Could you check a few things on this drawing? It's one solid part, dimensions in mm from its lowest x, y, z. Round coordinates to 2 decimals unless told otherwise and drop trailing zeros. Write each loop counter-clockwise with the first axis right and the second up, starting at its lowest first coordinate (ties: lowest second). Pieces come first, ordered by that corner, then holes. Notation, with made-up numbers: (-31.75, 82) - (23.25, 82) arc R23 ccw to (23.25, 111) - close; hole circle Ø3 at (-13, 81). An arc over 180 degrees is marked (long way). Put each result on its own line as item: value.
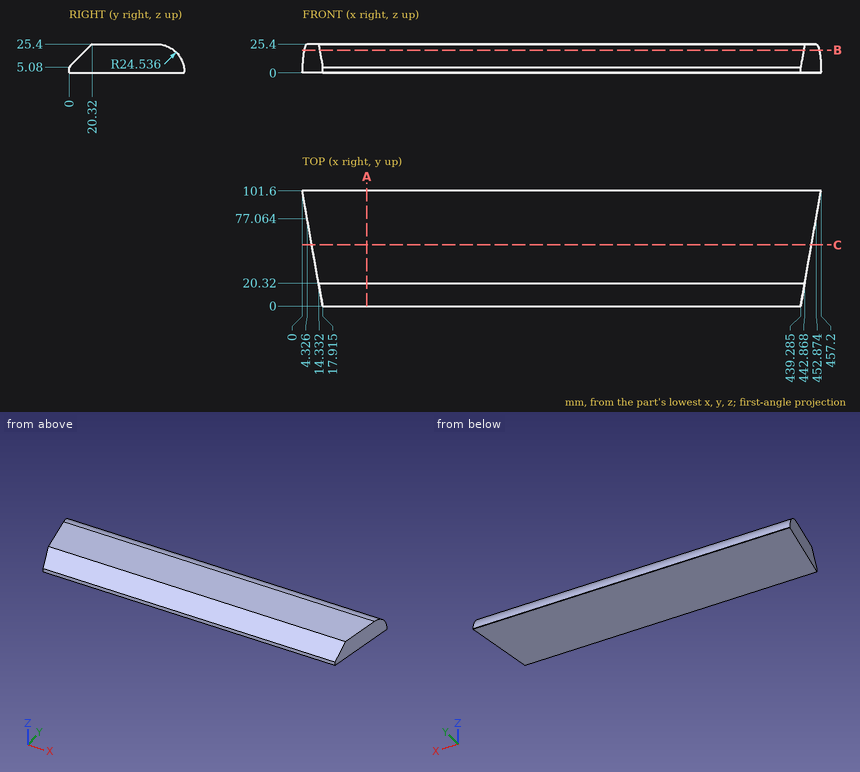
(1) Imagine slicing it at A-A, the plane x = 57. List the corners of the cut face in (y, z) for me.
Values found:
outline: (0, 0) - (101.6, 0) - (101.6, 0.86) arc R24.54 ccw to (77.06, 25.4) - (20.32, 25.4) - (0, 5.08) - close
(2) Imagine slicing it at B-B, the plane z = 20. List the corners of the cut face in (x, y) for me, then the cut area to 3 significant figures.
Values found:
outline: (1.62, 92.42) - (15.28, 14.92) - (441.92, 14.92) - (455.58, 92.42) - close
area: 34,100 mm^2
(3) Imagine slicing it at C-C, the plane y = 54. List the corners of the cut face in (x, z) for me, then the cut area to 3 significant figures.
Values found:
outline: (8.39, 0) - (448.81, 0) - (448.81, 25.4) - (8.39, 25.4) - close
area: 11,200 mm^2
(4) Please list where these lines run through material, in increasing order: probe 1 along Z at (x, y) = (196.5, 83); probe 2 along Y at (x, z) = (316.5, 7.5) (1 decimal); probe 3 along X at (y, z) = (80, 2). Write a range as from..to.
Values found:
probe 1: z = 0..24.67
probe 2: y = 2.4..100.7
probe 3: x = 3.81..453.39
(5) I'm going to push flat-ended pins straight in: pin 1 (4 mm diameter, centred on y = 71.5, z = 19.5, fed in from +X) (1 decimal); pin 2 (8 mm diameter, centred on y = 44.5, z = 12.5, fed in from -X); pin 3 (6 mm diameter, centred on y = 20, z = 12, fed in from -X). Where does each tip first touch, or does it pass through?
Values found:
pin 1: stops at x = 452.2
pin 2: stops at x = 9.36
pin 3: stops at x = 13.86
